CAD build for the part. Positions are in the model's coordinates, mm. Face numbers are marked on the shaded views. A direction names the side the tool comes from. Coordinates: 2 decimals unless noted, no trailing zeros. Write each loop counter-clockwise with the first axis right and the second up, starting at its lowest first coordinate (ties: lowest second). Pieces come first, ordered by that corner, then holes. Notation, with made-up numbers: (52.5, -38) - (72.5, -38) arc R8 ccw to (72.5, -29) - close; hole circle Ø2 at (-21, 8). An arc over 180 degrees is marked (long way). One line per question, with ' | ' between items. Start each with the question number.
1. Band-saw the part on A-A, the plane x = 0.55. Write the cut outline in (y, z).
2. Band-saw the part on C-C, the plane x = 2.75. Write the cut outline in (y, z).
3. Which spindle directions (+Z, -Z, +X, -X, +Y, -Y) get a long thin tool onto all of the face, cutting with end or side? Do the marked faces 1 and 2. Say none if no direction does.
4. Two-plate mould, pull along Y, no slides. Class the marked faces 3, 4 and 5: +Y half, -Y half, draft (parallel to the pull), parting line (faces both ways), or undercut.
5. Probe line 1 (Z direction, x = 1.95, y = -1.5); line 2 (Y direction, x = 1.4, z = 0.9); line 3 (X direction, y = -0.15, z = 0.15). List the from-to ranges inside material, lowest first.
6. Band-saw the part on B-B, the plane z = 0. Write the cut outline in (x, y).
7. Flat gauge pins, fed straight in: P1, Ø1, axis at y = 1.5, z = -2, coming from the +X side; P2, Ø0.8, axis at y = 0.5, z = 0, coming from the -X side. Where does each tip first touch, or does it go through?
from build123d import *

# Parameters (mm, degrees)
SKETCH1_W          = 4
SKETCH1_H          = 2.5
CUT_EXTRUDE1_DEPTH = 2
CHAMFER1_SIZE      = 0.75
CHAMFER2_SIZE      = 0.3
CHAMFER2_SIZE2     = 0.5


with BuildPart() as part:
    # Sketch1 → Revolve1 (revolve)
    with BuildSketch(Plane.XY):
        with Locations((2, 1.25)):
            Rectangle(SKETCH1_W, SKETCH1_H)
    revolve(axis=Axis((-0.394679187, 0, 0), (1, 0, 0)))

    # Sketch2 → Cut-Extrude1 (cut)
    with BuildSketch(Plane(origin=(0, 0, 0), x_dir=(0, 0, -1), z_dir=(1, 0, 0))):
        Polygon((-0.721687836, 1.25), (-1.443375673, 0), (-0.721687836, -1.25), (0.721687836, -1.25), (1.443375673, 0), (0.721687836, 1.25), align=None)
    extrude(amount=CUT_EXTRUDE1_DEPTH, mode=Mode.SUBTRACT)

    # Chamfer1
    chamfer1_edges = [part.edges().sort_by_distance(p)[0] for p in [
        (4, -2.5, 0),
    ]]
    chamfer(chamfer1_edges, length=CHAMFER1_SIZE)

    # Chamfer2
    chamfer2_edges = [part.edges().sort_by_distance(p)[0] for p in [
        (0, -2.5, 0),
    ]]
    chamfer2_side = [part.faces().sort_by_distance(p)[0] for p in [
        (1.625, -2.5, 0),
    ]]
    chamfer(chamfer2_edges, length=CHAMFER2_SIZE, length2=CHAMFER2_SIZE2, reference=chamfer2_side[0])


solid = part.part
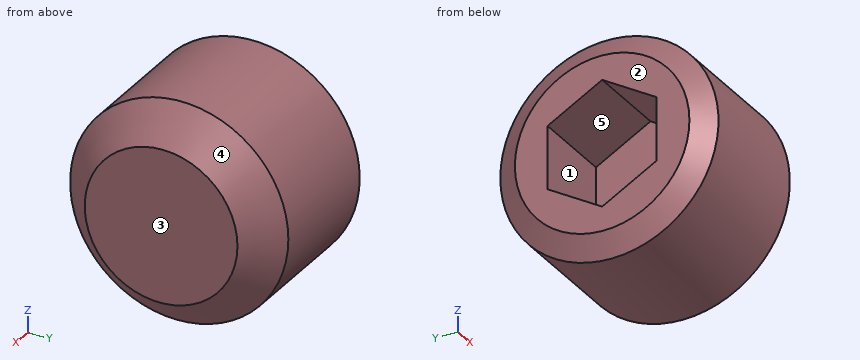
Filled in:
1) outline: circle Ø5 at (0, 0); hole (-1.25, -0.72) - (0, -1.44) - (1.25, -0.72) - (1.25, 0.72) - (0, 1.44) - (-1.25, 0.72) - close
2) outline: circle Ø5 at (0, 0)
3) face 1: -X | face 2: +Z, -Z, -X, +Y, -Y
4) face 3: draft | face 4: parting line | face 5: undercut
5) line 1: z = -2 to 2 | line 2: y = -2.33 to -0.94, 0.94 to 2.33 | line 3: x = 2 to 4
6) outline: (0, -2) - (0.3, -2.5) - (3.25, -2.5) - (4, -1.75) - (4, 1.75) - (3.25, 2.5) - (0.3, 2.5) - (0, 2) - (0, 1.25) - (2, 1.25) - (2, -1.25) - (0, -1.25) - close
7) P1: stops at x = 3.75 | P2: stops at x = 2
